Build history of the part. All positions in model axes, mm. A direction names the side the tool comes from. Coordinates: 2 decimals unless noted, no trailing zeros. One line per item, written item: value.
```python
from build123d import *

# Parameters (mm, degrees)
SKETCH1_R           = 3.556
SKETCH1_R_2         = 2.794
BOSS_EXTRUDE1_DEPTH = 10.16
SKETCH2_R           = 5.334
CUT_EXTRUDE1_DEPTH  = 3.81
CUT_EXTRUDE2_DEPTH  = 5.08
CHAMFER1_SIZE       = 3.81


with BuildPart() as part:
    # Sketch1 → Boss-Extrude1 (new body)
    with BuildSketch(Plane.XY):
        with BuildLine():
            Line((40.64, -38.735), (-40.64, -38.735))
            ThreePointArc((-40.64, -38.735), (-43.334076836, -37.619076836), (-44.45, -34.925))
            Line((-44.45, -34.925), (-44.45, 34.925))
            ThreePointArc((-44.45, 34.925), (-43.334076836, 37.619076836), (-40.64, 38.735))
            Line((-40.64, 38.735), (40.64, 38.735))
            ThreePointArc((40.64, 38.735), (43.334076836, 37.619076836), (44.45, 34.925))
            Line((44.45, 34.925), (44.45, -34.925))
            ThreePointArc((44.45, -34.925), (43.334076836, -37.619076836), (40.64, -38.735))
        make_face()
        with Locations((-34.671, -9.271)):
            Circle(SKETCH1_R, mode=Mode.SUBTRACT)
        with Locations((-34.671, -28.829)):
            Circle(SKETCH1_R, mode=Mode.SUBTRACT)
        with Locations((34.671, -9.271)):
            Circle(SKETCH1_R, mode=Mode.SUBTRACT)
        with Locations((34.671, -28.829)):
            Circle(SKETCH1_R, mode=Mode.SUBTRACT)
        with Locations((-19.939, 20.574)):
            Circle(SKETCH1_R_2, mode=Mode.SUBTRACT)
        with Locations(Location((19.939, 20.574, 0), (0, 0, 180))):
            Circle(SKETCH1_R_2, mode=Mode.SUBTRACT)
        with Locations((19.939, -20.574)):
            Circle(SKETCH1_R_2, mode=Mode.SUBTRACT)
        with Locations(Location((-19.939, -20.574, 0), (0, 0, 180))):
            Circle(SKETCH1_R_2, mode=Mode.SUBTRACT)
        with Locations((29.972, 9.906)):
            Circle(SKETCH1_R_2, mode=Mode.SUBTRACT)
        with Locations((-29.972, 9.906)):
            Circle(SKETCH1_R_2, mode=Mode.SUBTRACT)
    extrude(amount=BOSS_EXTRUDE1_DEPTH)

    # Sketch2 → Cut-Extrude1 (cut)
    with BuildSketch(Plane(origin=(0, 0, 0), x_dir=(-1, 0, 0), z_dir=(0, 0, -1))):
        with Locations((-19.939, 20.574)):
            Circle(SKETCH2_R)
        with Locations((19.939, -20.574)):
            Circle(SKETCH2_R)
        with Locations((-19.939, -20.574)):
            Circle(SKETCH2_R)
        with Locations((19.939, 20.574)):
            Circle(SKETCH2_R)
        with Locations((-29.972, 9.906)):
            Circle(SKETCH2_R)
        with Locations((29.972, 9.906)):
            Circle(SKETCH2_R)
    extrude(amount=-CUT_EXTRUDE1_DEPTH, mode=Mode.SUBTRACT)

    # Sketch3 → Cut-Extrude2 (cut)
    with BuildSketch(Plane.XY.offset(10.16)):
        Polygon((-31.738060633, -14.351), (-28.805121265, -9.271), (-31.738060633, -4.191), (-37.603939367, -4.191), (-40.536878735, -9.271), (-37.603939367, -14.351), align=None)
        Polygon((-31.738060633, -33.909), (-28.805121265, -28.829), (-31.738060633, -23.749), (-37.603939367, -23.749), (-40.536878735, -28.829), (-37.603939367, -33.909), align=None)
        Polygon((37.603939367, -33.909), (31.738060633, -33.909), (28.805121265, -28.829), (31.738060633, -23.749), (37.603939367, -23.749), (40.536878735, -28.829), align=None)
        Polygon((37.603939367, -14.351), (31.738060633, -14.351), (28.805121265, -9.271), (31.738060633, -4.191), (37.603939367, -4.191), (40.536878735, -9.271), align=None)
    extrude(amount=-CUT_EXTRUDE2_DEPTH, mode=Mode.SUBTRACT)

    # Chamfer1
    # the kernel refuses this chamfer: 3.81 mm, written as the material it takes off along each edge
    with BuildSketch(Plane(origin=(19.939, 20.574, 0), x_dir=(-1, 0, 0), z_dir=(0, -1, 0))) as chamfer1_piece_1_section:
        Polygon((5.334 + CHAMFER1_SIZE, 0), (5.334, -CHAMFER1_SIZE), (5.334, 0), align=None)
    chamfer1_piece_1 = revolve(axis=Axis((19.939, 20.574, 0), (0, 0, -1)), mode=Mode.PRIVATE)
    chamfer1_piece_1 = split(chamfer1_piece_1, bisect_by=Plane(origin=(27.18300283, 20.574, 3.81), z_dir=(0, 0, -1)), keep=Keep.TOP, mode=Mode.PRIVATE)
    add(chamfer1_piece_1, mode=Mode.SUBTRACT)
    with BuildSketch(Plane(origin=(-19.939, 20.574, 0), x_dir=(-1, 0, 0), z_dir=(0, -1, 0))) as chamfer1_piece_2_section:
        Polygon((5.334 + CHAMFER1_SIZE, 0), (5.334, -CHAMFER1_SIZE), (5.334, 0), align=None)
    chamfer1_piece_2 = revolve(axis=Axis((-19.939, 20.574, 0), (0, 0, -1)), mode=Mode.PRIVATE)
    chamfer1_piece_2 = split(chamfer1_piece_2, bisect_by=Plane(origin=(-12.694997174, 20.574, 3.81), z_dir=(0, 0, -1)), keep=Keep.TOP, mode=Mode.PRIVATE)
    add(chamfer1_piece_2, mode=Mode.SUBTRACT)
    with BuildSketch(Plane(origin=(-19.939, -20.574, 0), x_dir=(-1, 0, 0), z_dir=(0, -1, 0))) as chamfer1_piece_3_section:
        Polygon((5.334 + CHAMFER1_SIZE, 0), (5.334, -CHAMFER1_SIZE), (5.334, 0), align=None)
    chamfer1_piece_3 = revolve(axis=Axis((-19.939, -20.574, 0), (0, 0, -1)), mode=Mode.PRIVATE)
    chamfer1_piece_3 = split(chamfer1_piece_3, bisect_by=Plane(origin=(-12.694997169, -20.574, 3.81), z_dir=(0, 0, -1)), keep=Keep.TOP, mode=Mode.PRIVATE)
    add(chamfer1_piece_3, mode=Mode.SUBTRACT)
    with BuildSketch(Plane(origin=(19.939, -20.574, 0), x_dir=(-1, 0, 0), z_dir=(0, -1, 0))) as chamfer1_piece_4_section:
        Polygon((5.334 + CHAMFER1_SIZE, 0), (5.334, -CHAMFER1_SIZE), (5.334, 0), align=None)
    chamfer1_piece_4 = revolve(axis=Axis((19.939, -20.574, 0), (0, 0, -1)), mode=Mode.PRIVATE)
    chamfer1_piece_4 = split(chamfer1_piece_4, bisect_by=Plane(origin=(27.183002828, -20.574, 3.81), z_dir=(0, 0, -1)), keep=Keep.TOP, mode=Mode.PRIVATE)
    add(chamfer1_piece_4, mode=Mode.SUBTRACT)
    with BuildSketch(Plane(origin=(29.972, 9.906, 0), x_dir=(-1, 0, 0), z_dir=(0, -1, 0))) as chamfer1_piece_5_section:
        Polygon((5.334 + CHAMFER1_SIZE, 0), (5.334, -CHAMFER1_SIZE), (5.334, 0), align=None)
    chamfer1_piece_5 = revolve(axis=Axis((29.972, 9.906, 0), (0, 0, -1)), mode=Mode.PRIVATE)
    chamfer1_piece_5 = split(chamfer1_piece_5, bisect_by=Plane(origin=(37.216002826, 9.906, 3.81), z_dir=(0, 0, -1)), keep=Keep.TOP, mode=Mode.PRIVATE)
    add(chamfer1_piece_5, mode=Mode.SUBTRACT)
    with BuildSketch(Plane(origin=(-29.972, 9.906, 0), x_dir=(-1, 0, 0), z_dir=(0, -1, 0))) as chamfer1_piece_6_section:
        Polygon((5.334 + CHAMFER1_SIZE, 0), (5.334, -CHAMFER1_SIZE), (5.334, 0), align=None)
    chamfer1_piece_6 = revolve(axis=Axis((-29.972, 9.906, 0), (0, 0, -1)), mode=Mode.PRIVATE)
    chamfer1_piece_6 = split(chamfer1_piece_6, bisect_by=Plane(origin=(-22.727997169, 9.906, 3.81), z_dir=(0, 0, -1)), keep=Keep.TOP, mode=Mode.PRIVATE)
    add(chamfer1_piece_6, mode=Mode.SUBTRACT)


solid = part.part
```
Item 1: Tool access for faces 3 (the face through (1, 1, 10.16)), 4 (the face through (30.8, -9.2, 5.08)): list every direction of +Z, -Z, +X, -X, +Y, -Y with a clear straight run to the whole face (end or side of a thin tool).
Check result:
face 3: +Z, +X, -X, +Y, -Y
face 4: +Z
Item 2: Pull direction Y, two halves, no side cores. Call faces 1 (the face through (-44.45, 0, 5)), 2 (the face through (18.65, 23.053, 6.941)): released by +Y, released by -Y, zero draft, split by the parting line, or undercut.
Check result:
face 1: zero draft
face 2: undercut
Item 3: Probe probe 1 along X at (y, z) = (-9.5, 4.75); probe 2 along X at (y, z) = (-7.5, 5.25); probe 3 along Y at (x, z) = (19, 2.75) (3 decimals). List the from-to ranges inside material, lowest first. Write a range as from..to.
Check result:
probe 1: x = -44.45..-38.22, -31.12..31.12, 38.22..44.45
probe 2: x = -44.45..-39.51, -29.83..29.83, 39.51..44.45
probe 3: y = -38.735..-26.899, -14.249..14.249, 26.899..38.735
Item 4: Cut at A-A, the plane z = 1.25. Give the number of separate pieces and of enclosed holes in the cut face, then the cut area to 3 significant figures.
Check result:
separate pieces: 1
enclosed holes: 8
area: 5,550 mm^2
Item 5: Drop flat-ended pins along their axis: P1, Ø1.5, axis at x = 34.5, y = 11, coming from the -Z side; P2, Ø7.5, axis at x = 19.939, y = -20.574, coming from the -Z side. Give the stop position or say it passes through.
Check result:
P1: stops at z = 3.74
P2: stops at z = 3.81
